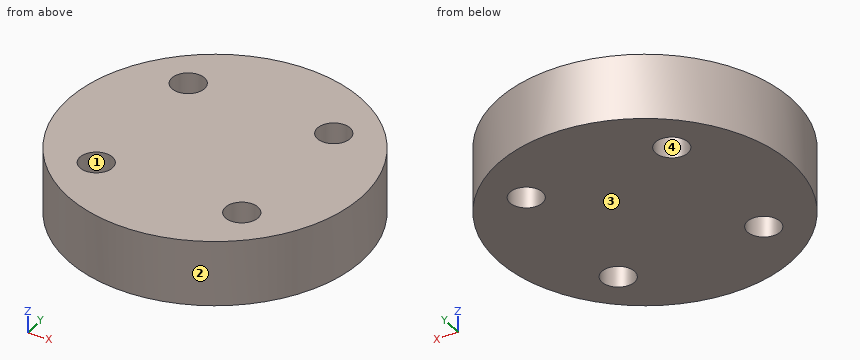
from build123d import *

# Parameters (mm, degrees)
CYLINDER970_R     = 1
CYLINDER970_DEPTH = 20
CYLINDER971_R     = 1
CYLINDER971_DEPTH = 20
CYLINDER965_R     = 1
CYLINDER965_DEPTH = 20
CYLINDER972_R     = 1
CYLINDER972_DEPTH = 20
CYLINDER978_R     = 9
CYLINDER978_DEPTH = 4


with BuildPart() as obj1:
    # Cylinder970 → Cylinder970 (new body)
    with BuildSketch(Plane(origin=(4.5, -4.5, -88), x_dir=(0, 1, 0), z_dir=(0, 0, 1))):
        Circle(CYLINDER970_R)
    extrude(amount=CYLINDER970_DEPTH)


with BuildPart() as obj2:
    # Cylinder971 → Cylinder971 (new body)
    with BuildSketch(Plane(origin=(4.5, 4.5, -88), x_dir=(-1, 0, 0), z_dir=(0, 0, 1))):
        Circle(CYLINDER971_R)
    extrude(amount=CYLINDER971_DEPTH)


with BuildPart() as obj3:
    # Cylinder965 → Cylinder965 (new body)
    with BuildSketch(Plane(origin=(-4.5, 4.5, -88), x_dir=(0, -1, 0), z_dir=(0, 0, 1))):
        Circle(CYLINDER965_R)
    extrude(amount=CYLINDER965_DEPTH)


with BuildPart() as compound808:
    # Cylinder972 → Cylinder972 (new body)
    with BuildSketch(Plane(origin=(-4.5, -4.5, -88), x_dir=(1, 0, 0), z_dir=(0, 0, 1))):
        Circle(CYLINDER972_R)
    extrude(amount=CYLINDER972_DEPTH)

    # Compound808: union obj1, obj2, obj3
    add(obj1.part)
    add(obj2.part)
    add(obj3.part)


with BuildPart() as compound808_1:
    # Compound808 placement: moved
    add(compound808.part.moved(Location((0, 0, 91))))


with BuildPart() as cut412:
    # Cylinder978 → Cylinder978 (new body)
    with BuildSketch(Plane.XY.offset(15)):
        Circle(CYLINDER978_R)
    extrude(amount=CYLINDER978_DEPTH)

    # Cut412: cut Compound808
    add(compound808_1.part, mode=Mode.SUBTRACT)


solid = cut412.part
Model file for the job. Use its own axes, mm. Face numbers are marked on the shaded views. Give positions to 0.01 mm unless a question says otherwise; leave off trailing zeros. Order: outer loops, then holes, each group sorted by start corner. A loop starts at its lowest first (then second) coordinate and runs counter-clockwise, first axis right, second up. Notation, with made-up numbers: (-24, 49.5) - (16, 49.5) arc R23 cw to (16, 65.5) - close; hole circle Ø2 at (82.25, -14.75). An arc over 180 degrees is marked (long way). Return JSON: item names as keys, results as strings.
1) Cut at B-B, the plane z = 16.25. Give the cut face in (x, y).
Geometry says:
{"outline": "circle Ø18 at (0, 0); hole circle Ø2 at (-4.5, -4.5); hole circle Ø2 at (-4.5, 4.5); hole circle Ø2 at (4.5, -4.5); hole circle Ø2 at (4.5, 4.5)"}
2) Probe line 1 (X direction, y = -4.25, z = 18.3); line 2 (Y direction, x = -4.5, z = 16.75); line 3 (X direction, y = -0.25, z = 18.15). List the from-to ranges inside material, lowest first. Write a range as from..to.
Geometry says:
{"line 1": "-7.93..-5.47, -3.53..3.53, 5.47..7.93", "line 2": "-7.79..-5.5, -3.5..3.5, 5.5..7.79", "line 3": "-9..9"}
3) Cut at D-D, the plane x = 2.25. Give the cut face in (y, z).
Geometry says:
{"outline": "(-8.71, 15) - (8.71, 15) - (8.71, 19) - (-8.71, 19) - close"}
4) Flat gauge pins, fed straight in: P1, Ø1.2, axis at x = 4.5, y = -4.5, coming from the +Z side; P2, Ø1.5, axis at y = 6, z = 18.5, coming from the -X side; P3, Ø1, axis at x = -5.5, z = 18, coming from the +Y side. Where does each tip first touch, or does it go through?
Geometry says:
{"P1": "through", "P2": "x = -7.31", "P3": "y = 7.48"}
5) Cut at A-A, the plane x = 4.5. Give the cut face in (y, z).
Geometry says:
{"outline": "(-7.79, 15) - (-5.5, 15) - (-5.5, 19) - (-7.79, 19) - close; (-3.5, 15) - (3.5, 15) - (3.5, 19) - (-3.5, 19) - close; (5.5, 15) - (7.79, 15) - (7.79, 19) - (5.5, 19) - close"}
6) Pull direction Y, two halves, no side cores. Call the marked faces 1, 2, 3 and 4: pulls with the +Y half, pulls with the -Y half, needs draft (parallel to the pull), parting line crosses it, or undercut.
Geometry says:
{"face 1": "undercut", "face 2": "parting line crosses it", "face 3": "needs draft", "face 4": "undercut"}
